Geometry check sheet. Reference: the model listing, model coordinates, mm. A direction names the side the tool comes from. Round coordinates to 2 decimals unless told otherwise and drop trailing zeros. Write each loop counter-clockwise with the first axis right and the second up, starting at its lowest first coordinate (ties: lowest second). Pieces come first, ordered by that corner, then holes. Notation, with made-up numbers: (58.5, 72.5) -> (113.5, 72.5) arc R34 cw to (113.5, 104.5) -> close; hole circle Ø5 at (-16.75, -8). An arc over 180 degrees is marked (long way). Return JSON: item names as keys, results as strings. Group by question number.
from build123d import *

# Parameters (mm, degrees)
F0_R     = 10.16
F1_DEPTH = 15.7734
F2_DEPTH = 40.2336
F3_DEPTH = 40.2346
F4_DEPTH = 25.4
F5_R     = 3.302


with BuildPart() as f1:
    # F0 (on Top) → F1 (new body)
    with BuildSketch(Plane.XY):
        with BuildLine():
            ThreePointArc((-26.278611, 28.126541), (-9.405233, 18.336262), (-2.746258, 0))
            ThreePointArc((-2.746258, 0), (-9.405233, -18.336262), (-26.278611, -28.126541))
            Line((-26.278611, -28.126541), (26.015507, -18.751028))
            ThreePointArc((26.015507, -18.751028), (3.603742, 0), (26.015507, 18.751028))
            Line((26.015507, 18.751028), (-26.278611, 28.126541))
        make_face()
        with BuildLine():
            ThreePointArc((-26.278611, -28.126541), (-9.405233, -18.336262), (-2.746258, 0))
            ThreePointArc((-2.746258, 0), (-9.405233, 18.336262), (-26.278611, 28.126541))
            ThreePointArc((-26.278611, 28.126541), (-59.896258, 0), (-26.278611, -28.126541))
        make_face()
        with BuildLine():
            ThreePointArc((-18.019436, -5.214805), (-45.602785, 0.413106), (-17.740244, 4.437195))
            Line((-17.740244, 4.437195), (-12.791958, 4.437195))
            Line((-12.791958, 4.437195), (-12.791958, -5.214805))
            Line((-12.791958, -5.214805), (-18.019436, -5.214805))
        make_face(mode=Mode.SUBTRACT)
        with BuildLine():
            ThreePointArc((-18.019436, -5.214805), (-17.28234, -2.653571), (-17.033758, 0))
            ThreePointArc((-17.033758, 0), (-17.211485, 2.246543), (-17.740244, 4.437195))
            Line((-17.740244, 4.437195), (-31.321258, 4.437195))
            Line((-31.321258, 4.437195), (-31.321258, -5.214805))
            Line((-31.321258, -5.214805), (-18.019436, -5.214805))
        make_face()
        with Locations((22.653742, 0)):
            Circle(F0_R)
        with BuildLine():
            Line((-31.321258, 4.437195), (-17.740244, 4.437195))
            ThreePointArc((-17.740244, 4.437195), (-45.602785, 0.413106), (-18.019436, -5.214805))
            Line((-18.019436, -5.214805), (-31.321258, -5.214805))
            Line((-31.321258, -5.214805), (-31.321258, 4.437195))
        make_face()
        with BuildLine():
            ThreePointArc((-17.740244, 4.437195), (-17.211485, 2.246543), (-17.033758, 0))
            ThreePointArc((-17.033758, 0), (-17.28234, -2.653571), (-18.019436, -5.214805))
            Line((-18.019436, -5.214805), (-12.791958, -5.214805))
            Line((-12.791958, -5.214805), (-12.791958, 4.437195))
            Line((-12.791958, 4.437195), (-17.740244, 4.437195))
        make_face()
        with BuildLine():
            ThreePointArc((41.703742, 0), (37.264425, 12.224174), (26.015507, 18.751028))
            ThreePointArc((26.015507, 18.751028), (3.603742, 0), (26.015507, -18.751028))
            ThreePointArc((26.015507, -18.751028), (37.264425, -12.224174), (41.703742, 0))
        make_face()
        with Locations((22.653742, 0)):
            Circle(F0_R, mode=Mode.SUBTRACT)
    extrude(amount=F1_DEPTH)

    # F0 (on Top) → F2 (join)
    with BuildSketch(Plane.XY):
        with BuildLine():
            ThreePointArc((-26.278611, -28.126541), (-9.405233, -18.336262), (-2.746258, 0))
            ThreePointArc((-2.746258, 0), (-9.405233, 18.336262), (-26.278611, 28.126541))
            ThreePointArc((-26.278611, 28.126541), (-59.896258, 0), (-26.278611, -28.126541))
        make_face()
        with BuildLine():
            ThreePointArc((-18.019436, -5.214805), (-45.602785, 0.413106), (-17.740244, 4.437195))
            Line((-17.740244, 4.437195), (-12.791958, 4.437195))
            Line((-12.791958, 4.437195), (-12.791958, -5.214805))
            Line((-12.791958, -5.214805), (-18.019436, -5.214805))
        make_face(mode=Mode.SUBTRACT)
    extrude(amount=F2_DEPTH)

    # F0 (on Top) → F3 (cut, through all)
    with BuildSketch(Plane.XY):
        with BuildLine():
            ThreePointArc((-18.019436, -5.214805), (-17.28234, -2.653571), (-17.033758, 0))
            ThreePointArc((-17.033758, 0), (-17.211485, 2.246543), (-17.740244, 4.437195))
            Line((-17.740244, 4.437195), (-31.321258, 4.437195))
            Line((-31.321258, 4.437195), (-31.321258, -5.214805))
            Line((-31.321258, -5.214805), (-18.019436, -5.214805))
        make_face()
        with BuildLine():
            ThreePointArc((-17.740244, 4.437195), (-17.211485, 2.246543), (-17.033758, 0))
            ThreePointArc((-17.033758, 0), (-17.28234, -2.653571), (-18.019436, -5.214805))
            Line((-18.019436, -5.214805), (-12.791958, -5.214805))
            Line((-12.791958, -5.214805), (-12.791958, 4.437195))
            Line((-12.791958, 4.437195), (-17.740244, 4.437195))
        make_face()
        with BuildLine():
            Line((-31.321258, 4.437195), (-17.740244, 4.437195))
            ThreePointArc((-17.740244, 4.437195), (-45.602785, 0.413106), (-18.019436, -5.214805))
            Line((-18.019436, -5.214805), (-31.321258, -5.214805))
            Line((-31.321258, -5.214805), (-31.321258, 4.437195))
        make_face()
    extrude(amount=F3_DEPTH, mode=Mode.SUBTRACT)

    # F0 (on Top) → F4 (cut)
    with BuildSketch(Plane.XY):
        with Locations((22.653742, 0)):
            Circle(F0_R)
    extrude(amount=F4_DEPTH, mode=Mode.SUBTRACT)

    # F5
    f5_edges = [f1.edges().sort_by_distance(p)[0] for p in [
        (-36.363905, 28.126541, 40.2336),
    ]]
    fillet(f5_edges, radius=F5_R)


solid = f1.part
1) Material ranges on probe 1 along X at (y, z) = (0, 27); probe 2 along Z at (x, y) = (-10.5, 22.5); probe 3 along X at (y, z) = (-1, 19.5), recorded low to high. Write a range as [from, to].
2) Mould release check, pull along Y, two halves, no side actions. Record for faces 1 (the face through (12.5, 0.4, 7.8)), 2 (the face through (0.235, 23.373, 7.776)), 3 (the face through (-20, -11, 40.234)), 4 (the face through (-0.498, -23.504, 7.776)): +Y half, -Y half, draft (parallel to the pull), parting line (faces both ways), or undercut.
3) Tool access check on faces 5 (the face through (-10, 0, 0)), 6 (the face through (-12.792, 0, 20)). Record the directions out of +Z, -Z, +X, -X, +Y, -Y that give a thin tool (end or side, any length) a straight path to the whole face; none if there is none.
4) Sectioned sample at C-C on x = 18.5. Enter the section's corners in (y, z), and give its area (3 significant figures).
5) Sectioned sample at A-A on x = 29.5. Enter the section's corners in (y, z).
6) Go/stop test with flat-tipped pins: P1, Ø2, axis at y = 12, z = 18.5, coming from the -X side; P2, Ø10, axis at y = -22.5, z = 18, coming from the -X side; P3, Ø2.5, axis at x = -15, z = 18.5, coming from the +Y side; P4, Ø23, axis at x = -31.32, y = 0, coming from the +Z side. Record where each tip stops, or that it passes through.
Evaluation:
{
 "1": {"probe 1": "x = [-59.9, -45.61], [-12.79, -2.75]", "probe 2": "z = [0, 15.77]", "probe 3": "x = [-59.88, -45.57], [-12.79, -2.76]"},
 "2": {"face 1": "undercut", "face 2": "+Y half", "face 3": "draft", "face 4": "-Y half"},
 "3": {"face 5": "-Z, +X, -X, +Y, -Y", "face 6": "+Z, -Z"},
 "4": {"outline": "(-20.1, 0) -> (-9.27, 0) -> (-9.27, 15.77) -> (-20.1, 15.77) -> close; (9.27, 0) -> (20.1, 0) -> (20.1, 15.77) -> (9.27, 15.77) -> close", "area": "342 mm2"},
 "5": {"outline": "(-17.78, 0) -> (-7.51, 0) -> (-7.51, 15.77) -> (-17.78, 15.77) -> close; (7.51, 0) -> (17.78, 0) -> (17.78, 15.77) -> (7.51, 15.77) -> close"},
 "6": {"P1": "stops at x = -57.69", "P2": "stops at x = -53.91", "P3": "stops at y = 24.28", "P4": "passes through"}
}
